Autodesk Inventor part; units mm, degrees
ref_plane "YZ Plane" through (0, 0, 0) normal (1, 0, 0) x (0, 1, 0)
ref_plane "XZ Plane" through (0, 0, 0) normal (0, 1, 0) x (-1, 0, 0)
ref_plane "XY Plane" through (0, 0, 0) normal (0, 0, 1) x (1, 0, 0)
sketch "Esboço1" plane through (0, 0, 0) normal (0, 0, 1) x (1, 0, 0)
  line L0 (60, -135) -> (-60, -135)
  line L1 (-60, -135) -> (-60, 135)
  line L2 (-60, 135) -> (60, 135)
  line L3 (60, 135) -> (60, -135)
  line L4 (60, -135) -> (-60, 135) construction
  line L5 (-60, -135) -> (60, 135) construction
  point P0 (0, 0)
  dimension "d0" = 120
  dimension "d1" = 270
extrude "Extrusão1" add sketch "Esboço1" along normal blind 3
sketch "Esboço3" plane through (60, -135, 0) normal (1, 0, 0) x (0, 0, -1)
  line L0 (0, 0) -> (-3, 0)
  line L1 (0, 0) -> (-3, 0)
  line L2 (-3, 0) -> (-3, 18.1)
  line L3 (-3, 18.1) -> (0, 18.1)
  line L4 (0, 18.1) -> (0, 0)
  line L5 (-3, 2.9) -> (0, 2.9)
  line L6 (-3, 48.1) -> (0, 48.1)
  line L7 (-3, 32.9) -> (0, 32.9)
  line L8 (-3, 78.1) -> (0, 78.1)
  line L9 (-3, 62.9) -> (0, 62.9)
  line L10 (-3, 108.1) -> (0, 108.1)
  line L11 (-3, 92.9) -> (0, 92.9)
  line L12 (-3, 138.1) -> (0, 138.1)
  line L13 (-3, 122.9) -> (0, 122.9)
  line L14 (-3, 168.1) -> (0, 168.1)
  line L15 (-3, 152.9) -> (0, 152.9)
  line L16 (-3, 198.1) -> (0, 198.1)
  line L17 (-3, 182.9) -> (0, 182.9)
  line L18 (-3, 228.1) -> (0, 228.1)
  line L19 (-3, 212.9) -> (0, 212.9)
  line L20 (-3, 258.1) -> (0, 258.1)
  line L21 (-3, 242.9) -> (0, 242.9)
  line L22 (-3, 288.1) -> (0, 288.1)
  line L23 (-3, 272.9) -> (0, 272.9)
  line L24 (-3, 0) -> (-3, 270)
  line L25 (0, 0) -> (0, 270)
  point P0 (0, 135)
  dimension "d13" = 18.1
  dimension "d14" = 3
  dimension "d38" = 2.9
  dimension "d41" = 30
extrude "Extrusão2" cut sketch "Esboço3" against normal blind 3 contours L0 L2 L5 L4 | L5 L2 L3 L4 | L7 L24 L6 L25 | L9 L24 L8 L25 | L11 L24 L10 L25 | L13 L24 L12 L25 | L15 L24 L14 L25 | L17 L24 L16 L25 | L19 L24 L18 L25 | L21 L24 L20 L25
sketch "Esboço5" plane through (57, -135, 0) normal (0, -1, 0) x (1, 0, 0)
  line L0 (-117, 0) -> (0, 0)
  line L1 (-114, 3) -> (-98.8, 3)
  line L2 (-98.8, 3) -> (-98.8, 0)
  line L3 (-98.8, 0) -> (-114, 0)
  line L4 (-114, 0) -> (-114, 3)
  line L5 (-84, 3) -> (-68.8, 3)
  line L6 (-68.8, 3) -> (-68.8, 0)
  line L7 (-68.8, 0) -> (-84, 0)
  line L8 (-84, 0) -> (-84, 3)
  line L9 (-54, 3) -> (-38.8, 3)
  line L10 (-38.8, 3) -> (-38.8, 0)
  line L11 (-38.8, 0) -> (-54, 0)
  line L12 (-54, 0) -> (-54, 3)
  line L13 (-24, 3) -> (-8.8, 3)
  line L14 (-8.8, 3) -> (-8.8, 0)
  line L15 (-8.8, 0) -> (-24, 0)
  line L16 (-24, 0) -> (-24, 3)
  line L17 (-117, 0) -> (-117, 3)
  point P0 (-57, 0)
  point P1 (-24, 0)
  point P2 (-54, 0)
  point P3 (-84, 0)
  point P4 (-117, 1.5)
  point P5 (-114, 1.5)
  dimension "d26" = 15.2
  dimension "d29" = 30
  dimension "d56" = 3
extrude "Extrusão4" cut sketch "Esboço5" against normal blind 3
sketch "Esboço7" plane through (-60, -135, 0) normal (-1, 0, 0) x (0, 0, 1)
  line L0 (3, 18.1) -> (0, 18.1)
  line L1 (3, 0) -> (3, 18.1)
  line L2 (0, 18.1) -> (0, 0)
  line L3 (0, 32.9) -> (3, 32.9)
  line L4 (3, 270) -> (3, 0)
  line L5 (0, 270) -> (0, 0)
  line L6 (0, 32.9) -> (3, 32.9)
  line L7 (0, 18.1) -> (3, 18.1)
  line L8 (0, 48.1) -> (3, 48.1)
  line L9 (0, 62.9) -> (3, 62.9)
  line L10 (0, 78.1) -> (3, 78.1)
  line L11 (0, 92.9) -> (3, 92.9)
  line L12 (0, 108.1) -> (3, 108.1)
  line L13 (0, 122.9) -> (3, 122.9)
  line L14 (0, 138.1) -> (3, 138.1)
  line L15 (0, 152.9) -> (3, 152.9)
  line L16 (0, 168.1) -> (3, 168.1)
  line L17 (0, 182.9) -> (3, 182.9)
  line L18 (0, 198.1) -> (3, 198.1)
  line L19 (0, 212.9) -> (3, 212.9)
  line L20 (0, 228.1) -> (3, 228.1)
  line L21 (0, 242.9) -> (3, 242.9)
  line L22 (0, 258.1) -> (3, 258.1)
  line L23 (0, 272.9) -> (3, 272.9)
  line L24 (0, 288.1) -> (3, 288.1)
  line L25 (0, 302.9) -> (3, 302.9)
  line L26 (3, 0) -> (0, 0)
  line L27 (0, 0) -> (0, 270)
  line L28 (0, 270) -> (3, 270)
  line L29 (3, 270) -> (3, 0)
  point P0 (0, 135)
  point P1 (3, 258.1)
  point P2 (0, 258.1)
  point P3 (0, 242.9)
  point P4 (3, 242.9)
  point P5 (3, 228.1)
  point P6 (0, 228.1)
  point P7 (0, 212.9)
  point P8 (3, 212.9)
  point P9 (3, 198.1)
  point P10 (0, 198.1)
  point P11 (0, 182.9)
  point P12 (3, 182.9)
  point P13 (3, 168.1)
  point P14 (0, 168.1)
  point P15 (0, 152.9)
  point P16 (3, 152.9)
  point P17 (3, 138.1)
  point P18 (0, 138.1)
  point P19 (0, 122.9)
  point P20 (3, 122.9)
  point P21 (3, 108.1)
  point P22 (0, 108.1)
  point P23 (0, 92.9)
  point P24 (3, 92.9)
  point P25 (3, 78.1)
  point P26 (0, 78.1)
  point P27 (0, 62.9)
  point P28 (3, 62.9)
  point P29 (3, 48.1)
  point P30 (0, 48.1)
  dimension "d49" = 30
extrude "Extrusão5" cut sketch "Esboço7" against normal blind 3 contours L1 L26 L2 L0 | L3 L5 L8 L4 | L9 L5 L10 L4 | L11 L5 L12 L4 | L13 L5 L14 L4 | L15 L5 L16 L4 | L17 L5 L18 L4 | L19 L5 L20 L4 | L21 L5 L22 L4
sketch "Esboço8" plane through (0, 0, 0) normal (0, 0, -1) x (-1, 0, 0)
  line L0 (-57, -86.9) -> (-60, -86.9) construction
  line L1 (-60, -86.9) -> (-60, -72.1) construction
  line L2 (-60, -72.1) -> (-57, -72.1) construction
  line L3 (-57, -72.1) -> (-57, -56.9) construction
  line L4 (-57, -56.9) -> (-60, -56.9) construction
  line L5 (-60, -56.9) -> (-60, -42.1) construction
  line L6 (-60, -42.1) -> (-57, -42.1) construction
  line L7 (-57, -42.1) -> (-57, -26.9) construction
  line L8 (-57, -26.9) -> (-60, -26.9) construction
  line L9 (-60, -26.9) -> (-60, -12.1) construction
  line L10 (-60, -12.1) -> (-57, -12.1) construction
  line L11 (-57, -12.1) -> (-57, 3.1) construction
  line L12 (-57, 3.1) -> (-60, 3.1) construction
  line L13 (-60, 3.1) -> (-60, 17.9) construction
  line L14 (-60, 17.9) -> (-57, 17.9) construction
  line L15 (-57, 17.9) -> (-57, 33.1) construction
  line L16 (-57, 33.1) -> (-60, 33.1) construction
  line L17 (-60, 33.1) -> (-60, 47.9) construction
  line L18 (-60, 47.9) -> (-57, 47.9) construction
  line L19 (-57, 47.9) -> (-57, 63.1) construction
  line L20 (-57, 63.1) -> (-60, 63.1) construction
  line L21 (-60, 63.1) -> (-60, 77.9) construction
  line L22 (-60, 77.9) -> (-57, 77.9) construction
  line L23 (-57, 77.9) -> (-57, 93.1) construction
  line L24 (-57, 93.1) -> (-60, 93.1) construction
  line L25 (-60, 93.1) -> (-60, 107.9) construction
  line L26 (-60, 107.9) -> (-57, 107.9) construction
  line L27 (-57, 107.9) -> (-57, 123.1) construction
  line L28 (-57, 123.1) -> (-60, 123.1) construction
  line L29 (-60, 123.1) -> (-60, 135) construction
  line L30 (-60, 135) -> (60, 135) construction
  line L31 (60, 135) -> (60, 123.1) construction
  line L32 (60, 123.1) -> (57, 123.1) construction
  line L33 (57, 123.1) -> (57, 107.9) construction
  line L34 (57, 107.9) -> (60, 107.9) construction
  line L35 (60, 107.9) -> (60, 93.1) construction
  line L36 (60, 93.1) -> (57, 93.1) construction
  line L37 (57, 93.1) -> (57, 77.9) construction
  line L38 (57, 77.9) -> (60, 77.9) construction
  line L39 (60, 77.9) -> (60, 63.1) construction
  line L40 (60, 63.1) -> (57, 63.1) construction
  line L41 (57, 63.1) -> (57, 47.9) construction
  line L42 (57, 47.9) -> (60, 47.9) construction
  line L43 (60, 47.9) -> (60, 33.1) construction
  line L44 (60, 33.1) -> (57, 33.1) construction
  line L45 (57, 33.1) -> (57, 17.9) construction
  line L46 (57, 17.9) -> (60, 17.9) construction
  line L47 (60, 17.9) -> (60, 3.1) construction
  line L48 (60, 3.1) -> (57, 3.1) construction
  line L49 (57, 3.1) -> (57, -12.1) construction
  line L50 (57, -12.1) -> (60, -12.1) construction
  line L51 (60, -12.1) -> (60, -26.9) construction
  line L52 (60, -26.9) -> (57, -26.9) construction
  line L53 (57, -26.9) -> (57, -42.1) construction
  line L54 (57, -42.1) -> (60, -42.1) construction
  line L55 (60, -42.1) -> (60, -56.9) construction
  line L56 (60, -56.9) -> (57, -56.9) construction
  line L57 (57, -56.9) -> (57, -72.1) construction
  line L58 (57, -72.1) -> (60, -72.1) construction
  line L59 (60, -72.1) -> (60, -86.9) construction
  line L60 (60, -86.9) -> (57, -86.9) construction
  line L61 (57, -86.9) -> (57, -102.1) construction
  line L62 (57, -102.1) -> (60, -102.1) construction
  line L63 (60, -102.1) -> (60, -116.9) construction
  line L64 (60, -116.9) -> (57, -116.9) construction
  line L65 (57, -116.9) -> (57, -132) construction
  line L66 (57, -132) -> (41.8, -132) construction
  line L67 (41.8, -132) -> (41.8, -135) construction
  line L68 (41.8, -135) -> (27, -135) construction
  line L69 (27, -135) -> (27, -132) construction
  line L70 (27, -132) -> (11.8, -132) construction
  line L71 (11.8, -132) -> (11.8, -135) construction
  line L72 (11.8, -135) -> (-3, -135) construction
  line L73 (-3, -135) -> (-3, -132) construction
  line L74 (-3, -132) -> (-18.2, -132) construction
  line L75 (-18.2, -132) -> (-18.2, -135) construction
  line L76 (-18.2, -135) -> (-33, -135) construction
  line L77 (-33, -135) -> (-33, -132) construction
  line L78 (-33, -132) -> (-48.2, -132) construction
  line L79 (-48.2, -132) -> (-48.2, -135) construction
  line L80 (-48.2, -135) -> (-57, -135) construction
  line L81 (-57, -135) -> (-57, -116.9) construction
  line L82 (-57, -116.9) -> (-60, -116.9) construction
  line L83 (-60, -116.9) -> (-60, -102.1) construction
  line L84 (-60, -102.1) -> (-57, -102.1) construction
  line L85 (-57, -102.1) -> (-57, -86.9) construction
  ellipse E0 centre (-55.4, 11.3042) end of major axis (-55.4, 8.4758) minor radius 2 (-57.4, 11.3042) -> (-57.1743, 9.9988) ccw
  line L86 (-57.1743, 9.9988) -> (59.4, 9.9988)
  line L87 (59.4, 127.5) -> (59.4, 9.9988)
  line L88 (-57.4, 127.5) -> (59.4, 127.5)
  line L89 (-57.4, 127.5) -> (-57.4, 11.3042)
  ellipse E1 centre (-56.5, 121.6939) end of major axis (-56.5, 127.5415) minor radius 2 (-54.5, 121.6939) -> (-55.7002, 127.0537) ccw
  line L90 (-55.7002, 127.0537) -> (55.7002, 127.0537)
  ellipse E2 centre (56.5, 121.6939) end of major axis (56.5, 127.5415) minor radius 2 (55.7002, 127.0537) -> (54.5, 121.6939) ccw
  line L91 (54.5, 121.6939) -> (54.5, 105.9054)
  line L92 (54.5, 105.9054) -> (49.5, 105.9054) construction
  line L93 (49.5, 105.9054) -> (49.5, 116.4119) construction
  line L94 (49.5, 116.4119) -> (-49.5, 116.4119) construction
  line L95 (-49.5, 116.4119) -> (-49.5, 105.9054) construction
  line L96 (-49.5, 105.9054) -> (-54.5, 105.9054) construction
  line L97 (-54.5, 105.9054) -> (-54.5, 121.6939)
  circle A0 centre (-50, 132) radius 1.5
  circle A1 centre (0, 132) radius 1.5
  circle A2 centre (50, 132) radius 1.5
  line L98 (60, 7.3988) -> (-60, 7.3988)
  line L99 (-60, 7.3988) -> (-60, 136)
  line L100 (-60, 136) -> (60, 136)
  line L101 (60, 136) -> (60, 7.3988)
  line L102 (-60, 7.3988) -> (60, 7.3988)
  line L103 (60, 7.3988) -> (60, 15.3988)
  line L104 (60, 15.3988) -> (-60, 15.3988)
  line L105 (-60, 15.3988) -> (-60, 7.3988)
  line L106 (-60, 11.3988) -> (60, 11.3988) construction
  circle A3 centre (0, 11.3988) radius 1.6
  circle A4 centre (-50, 11.3988) radius 1.6
  circle A5 centre (50, 11.3988) radius 1.6
  line L107 (54.5, 66.3189) -> (54.5, 124.5798)
  line L108 (-54.5, 124.5798) -> (-54.5, 66.3189)
  line L109 (-60, 136) -> (60, 136)
  line L110 (-60, 135) -> (60, 135)
  line L111 (-54.7, 15.3988) -> (-54.7, 127.5)
  line L112 (54.7, 127.5) -> (54.7, 15.3988)
  point P0 (-60, 49.3988)
  point P1 (54.7, 127.0537)
  point P2 (-54.7, 127.0537)
  point P3 (54.7, 124.2429)
  point P4 (-54.7, 124.2429)
  point P5 (-55.6594, 127)
  point P6 (55.6594, 127)
  point P7 (-49.2254, 9.9988)
  point P8 (-50.7746, 9.9988)
  point P9 (0.7746, 9.9988)
  point P10 (-0.7746, 9.9988)
  point P11 (50.7746, 9.9988)
  point P12 (49.2254, 9.9988)
  dimension "d91" = 8
  dimension "d92" = 3.2
  dimension "d93" = 3.2
  dimension "d94" = 3.2
  dimension "d95" = 1
  dimension "d96" = 0.2
  dimension "d97" = 0.2
  dimension "d101" = 7.5
extrude "Extrusão6" cut sketch "Esboço8" against normal up to surface (3 mm away) contours A4 L86 | L86 A4 | L111 L90 L112 L104 | L88 L112 L90 L111 | A3 L86 | L86 A3 | A5 L86 | L86 A5 | A0 | A1 | A2
fillet "Arredondamento1" radius 5 2 edges at (54.7, 15.3988, 1.5) (-54.7, 15.3988, 1.5)
sketch "Esboço9" plane through (0, 0, 0) normal (0, 0, -1) x (-1, 0, 0)
  circle A0 centre (0, -59.8006) radius 26
  line L0 (49.7, 15.3988) -> (-49.7, 15.3988)
  line L1 (0, 15.3988) -> (0, -135) construction
  line L2 (11.8, -135) -> (-3, -135)
  point P0 (0, 0)
  point P1 (0, -59.8006)
  dimension "d102" = 52
extrude "Extrusão7" cut sketch "Esboço9" against normal up to surface (3 mm away)
equation "\"d14\" = d4"
equation "\"d93\" = d92"
equation "\"d94\" = d92"
properties part number "frente"
Part model, mm, in its own coordinate system. A direction names the side the tool comes from. Give positions to 0.01 mm unless a question says otherwise; leave off trailing zeros. Order: outer loops, then holes, each group sorted by start corner. A loop starts at its lowest first (then second) coordinate and runs counter-clockwise, first axis right, second up. Notation, with made-up numbers: (4.25, 60) - (50.25, 60) arc R13 ccw to (50.25, 77) - close; hole circle Ø9 at (2.5, 18.25). An arc over 180 degrees is marked (long way). Use a Markdown table: item, result.
1) Probe L1, parallel to X at y = 132, z = 0.7; L2, parallel to X at y = 53, z = 0.7; L3, parallel to X at y = 36, z = 1.25. List the from-to ranges inside material, lowest first. Write a range as from..to.
Checked values:
| item | result |
|---|---|
| L1 | -60..-51.5, -48.5..-1.5, 1.5..48.5, 51.5..60 |
| L2 | -57..-54.7, 54.7..57 |
| L3 | -60..-54.7, 54.7..60 |
2) Saw through at C-C on y = -48. List the corners of the cut face in (x, z).
Checked values:
| item | result |
|---|---|
| outline | (-60, 0) - (-23.17, 0) - (-23.17, 3) - (-60, 3) - close; (23.17, 0) - (60, 0) - (60, 3) - (23.17, 3) - close |
3) Saw through at B-B on x = -19. List the corners of the cut face in (y, z).
Checked values:
| item | result |
|---|---|
| outline | (-132, 0) - (-77.55, 0) - (-77.55, 3) - (-132, 3) - close; (-42.05, 0) - (15.4, 0) - (15.4, 3) - (-42.05, 3) - close; (127.5, 0) - (135, 0) - (135, 3) - (127.5, 3) - close |
4) Two-plate mould, pull along X, no slides. Class faces 3 (the cylindrical face through (5.64, -85.18, 1.48)), 4 (the flat face through (-28, -58, 3)): +X half, -X half, draft (parallel to the pull), parting line (faces both ways), or undercut.
Checked values:
| item | result |
|---|---|
| face 3 | undercut |
| face 4 | draft |
5) Flat gauge pins, fed straight in: P1, Ø0.9, axis at x = -59, z = 1, coming from the -Y side; P2, Ø1.5, axis at y = -134, z = 1, coming from the +X side; P3, Ø1.5, axis at x = -22.5, y = 1, coming from the -Z side. Where does each tip first touch, or does it go through?
Checked values:
| item | result |
|---|---|
| P1 | y = -116.9 |
| P2 | x = 57 |
| P3 | z = 0 |
6) Saw through at D-D on z = 2.1. Count the separate pieces of the cut face and the enclosed holes in it, plus the area to 3 significant figures.
Checked values:
| item | result |
|---|---|
| separate pieces | 1 |
| enclosed holes | 8 |
| area | 17,000 mm² |
7) Saw through at A-A on y = 113. List the corners of the cut face in (x, z), plus the area to 3 significant figures.
Checked values:
| item | result |
|---|---|
| outline | (-57, 0) - (-54.7, 0) - (-54.7, 3) - (-57, 3) - close; (54.7, 0) - (57, 0) - (57, 3) - (54.7, 3) - close |
| area | 13.8 mm² |
8) 3-axis set-ups, long thin cutter, end or side, ignore diameter. For faces 1 (the flat face through (-28, -58, 0)), 2 (the cylindrical face through (53.196, 16.825, 1.521)): which of +Z, -Z, +X, -X, +Y, -Y reach the whole face in a straight line?
Checked values:
| item | result |
|---|---|
| face 1 | -Z, +X, -X, +Y, -Y |
| face 2 | +Z, -Z |
